CAD build for the part. Positions are in the model's coordinates, mm. A direction names the side the tool comes from. Give positions to 0.01 mm unless a question says otherwise; leave off trailing zeros. Write each loop counter-clockwise with the first axis right and the second up, starting at its lowest first coordinate (ties: lowest second). Pieces come first, ordered by that corner, then holes. Notation, with made-up numbers: M -14,44.25 L 8,44.25 A32 cw 8,74.25 Z; hole C 35.5,77.5 d8. An arc over 180 degrees is marked long. One line per question, with ' | ' between items. Start each with the question number.
1. Which spindle directions (+Z, -Z, +X, -X, +Y, -Y) get a long thin tool onto all of the face, cutting with end or side? Do faces 1 (the face through (0.7, 29.4, 0)), 2 (the face through (-5, 49, 5)), 3 (the face through (6, 1, 5)). Say none if no direction does.
2. Wall check: L1, parallel to X at y = 33.5, z = 8.5; L2, parallel to Y at x = -4.75, z = 6. Give the ranges that are in metal, low to high.
3. Cut at A-A, the plane z = 2.25. Write the cut outline in (x, y), then the cut area to 3 significant figures.
4. Cut at B-B, the plane x = -4.75. Write the cut outline in (y, z).
5. Flat gauge pins, fed straight in: pin 1 (4 mm diameter, centred on y = 44.5, z = 6.5, fed in from -X); pin 2 (5.5 mm diameter, centred on x = -6, z = 6.5, fed in from -Y); pin 3 (1.5 mm diameter, centred on y = 21, z = 2.5, fed in from +X); pin 4 (8 mm diameter, centred on x = 0, y = 12, fed in from -Z). Where does each tip first touch, or does it go through?
6. Cut at C-C, the plane y = 45. Write the cut outline in (x, z).
```python
from build123d import *

# Parameters (mm, degrees)
F1_DEPTH = 9.5
F2_R     = 1


with BuildPart() as f1:
    # F0 (on Top) → F1 (new body)
    with BuildSketch(Plane.XY):
        Polygon((-2.12132, 49), (0, 49), (0, 46.87868), (0, 2.12132), (1, 1.12132), (1, 3.12132), (1, 51), (-7, 51), (-7, 49), align=None)
        Polygon((0, 46.87868), (0, 49), (-2.12132, 49), align=None)
        Polygon((1.12132, 1), (1, 1.12132), (1, 1), align=None)
        Polygon((1, 3.12132), (1, 1.12132), (1.12132, 1), (3.12132, 1), align=None)
        Polygon((3.12132, 1), (1.12132, 1), (2.12132, 0), (9.5, 0), (9.5, 1), align=None)
    extrude(amount=F1_DEPTH)

    # F2
    f2_edges = [f1.edges().sort_by_distance(p)[0] for p in [
        (9.5, 0.5, 9.5),
        (9.5, 0.5, 0),
    ]]
    fillet(f2_edges, radius=F2_R)


solid = f1.part
```
Here are the results:
1) face 1: -Z, +X, -X, +Y, -Y | face 2: +Z, -Z, -X, -Y | face 3: +Z, -Z, +X, +Y
2) L1: 0 to 1 | L2: 49 to 51
3) outline: M -7,49 L -2.12,49 L 0,46.88 L 0,2.12 L 1,1.12 L 1,1 L 1.12,1 L 2.12,0 L 9.5,0 L 9.5,1 L 3.12,1 L 1,3.12 L 1,51 L -7,51 Z | area: 75.8 mm^2
4) outline: M 49,0 L 51,0 L 51,9.5 L 49,9.5 Z
5) pin 1: x = 0 | pin 2: y = 49 | pin 3: x = 1 | pin 4: z = 0
6) outline: M 0,0 L 1,0 L 1,9.5 L 0,9.5 Z
